Design review of the part built by this model. Coordinates are the model's own, in mm. Give positions to 0.01 mm unless a question says otherwise; leave off trailing zeros. Loops run counter-clockwise (first coordinate to the right, second up) from the corner with the lowest first, then second, coordinate; pieces in that order, holes last.
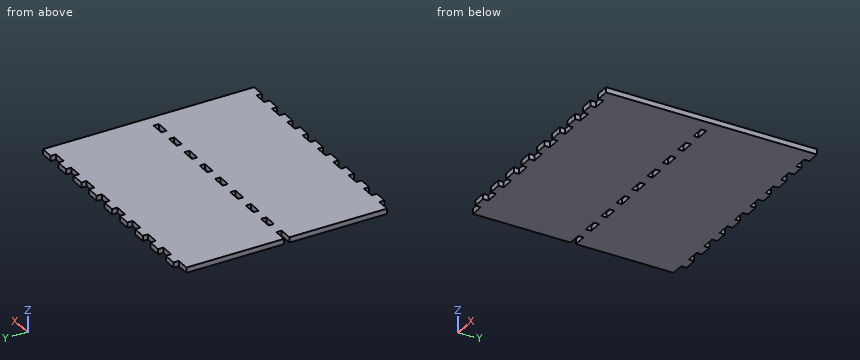
from build123d import *

# Parameters (mm, degrees)
F1_DEPTH = 6
F2_W     = 15
F2_H     = 3
F3_DEPTH = 6.001


with BuildPart() as f1:
    # F0 (on Top) → F1 (new body)
    with BuildSketch(Plane.XY):
        Polygon((15, 6), (15, 0), (30, 0), (30, 6), (45, 6), (45, 0), (60, 0), (60, 6), (75, 6), (75, 0), (90, 0), (90, 6), (105, 6), (105, 0), (120, 0), (120, 6), (135, 6), (135, 0), (150, 0), (150, 6), (165, 6), (165, 0), (180, 0), (180, 6), (195, 6), (195, 0), (210, 0), (210, 6), (225, 6), (225, 0), (240, 0), (240, 6), (255, 6), (255, 0), (270, 0), (270, 240), (255, 240), (255, 234), (240, 234), (240, 240), (225, 240), (225, 234), (210, 234), (210, 240), (195, 240), (195, 234), (180, 234), (180, 240), (165, 240), (165, 234), (150, 234), (150, 240), (135, 240), (135, 234), (120, 234), (120, 240), (105, 240), (105, 234), (90, 234), (90, 240), (75, 240), (75, 234), (60, 234), (60, 240), (45, 240), (45, 234), (30, 234), (30, 240), (15, 240), (15, 234), (0, 234), (0, 6), align=None)
    extrude(amount=F1_DEPTH)

    # F2 (on face) → F3 (cut, through all)
    with BuildSketch(Plane.XY.offset(6)):
        with Locations((7.5, 121.5)):
            Rectangle(F2_W, F2_H)
        with Locations((7.5, 118.5)):
            Rectangle(F2_W, F2_H)
        with Locations((37.5, 121.5)):
            Rectangle(F2_W, F2_H)
        with Locations((37.5, 118.5)):
            Rectangle(F2_W, F2_H)
        with Locations((67.5, 121.5)):
            Rectangle(F2_W, F2_H)
        with Locations((67.5, 118.5)):
            Rectangle(F2_W, F2_H)
        with Locations((97.5, 121.5)):
            Rectangle(F2_W, F2_H)
        with Locations((97.5, 118.5)):
            Rectangle(F2_W, F2_H)
        with Locations((127.5, 121.5)):
            Rectangle(F2_W, F2_H)
        with Locations((127.5, 118.5)):
            Rectangle(F2_W, F2_H)
        with Locations((157.5, 121.5)):
            Rectangle(F2_W, F2_H)
        with Locations((157.5, 118.5)):
            Rectangle(F2_W, F2_H)
        with Locations((187.5, 121.5)):
            Rectangle(F2_W, F2_H)
        with Locations((187.5, 118.5)):
            Rectangle(F2_W, F2_H)
        with Locations((247.5, 121.5)):
            Rectangle(F2_W, F2_H)
        with Locations((247.5, 118.5)):
            Rectangle(F2_W, F2_H)
        with Locations((217.5, 118.5)):
            Rectangle(F2_W, F2_H)
        with Locations((217.5, 121.5)):
            Rectangle(F2_W, F2_H)
    extrude(amount=-F3_DEPTH, mode=Mode.SUBTRACT)


solid = f1.part
Q1. Insertion check: pin 1 (3 mm diameter, centred on y = 237, z = 2, fed in from -X); pin 2 (3 mm diameter, centred on x = 69.5, z = 3, fed in from +Y); pin 3 (1.8 mm diameter, centred on x = 246, z = 2, fed in from -Y). Each pin has a flat end and moves straight along its axis. Give the tip position at first contact, or say it passes through.
Results:
pin 1: stops at x = 15
pin 2: stops at y = 234
pin 3: stops at y = 6
Q2. Take a section at A-A (x = 249). Give the boundary of the cut face in (y, z), plus the area to 3 significant figures.
Results:
outline: (6, 0) - (117, 0) - (117, 6) - (6, 6) - close; (123, 0) - (234, 0) - (234, 6) - (123, 6) - close
area: 1,330 mm2
Q3. Take a section at B-B (z = 2.1). Give the number of separate pieces and of enclosed holes in the cut face, plus the area to 3 significant figures.
Results:
separate pieces: 1
enclosed holes: 8
area: 62,400 mm2
Q4. Wall thickness on line 1 (Y direction, x = 42.5, z = 0.8): over which ranges is the line inside the solid? List them lowest first.
Results:
line 1: y = 6 to 117, 123 to 234
